Source: three-view drawing plus pictorial views. Frame: mm from the lowest corner of the part. Give positions to 0.01 mm unless a question says otherwise; leave off trailing zeros. Write each loop counter-clockwise with the first axis right and the second up, starting at its lowest first coordinate (ties: lowest second). Pieces come first, ordered by that corner, then holes. Notation, with made-up numbers: M 10.5,-17 L 28.5,-17 A28 ccw 28.5,21 Z; hole C 64,44.5 d2. An arc over 180 degrees is marked long. Return JSON: item names as keys, results as strings.
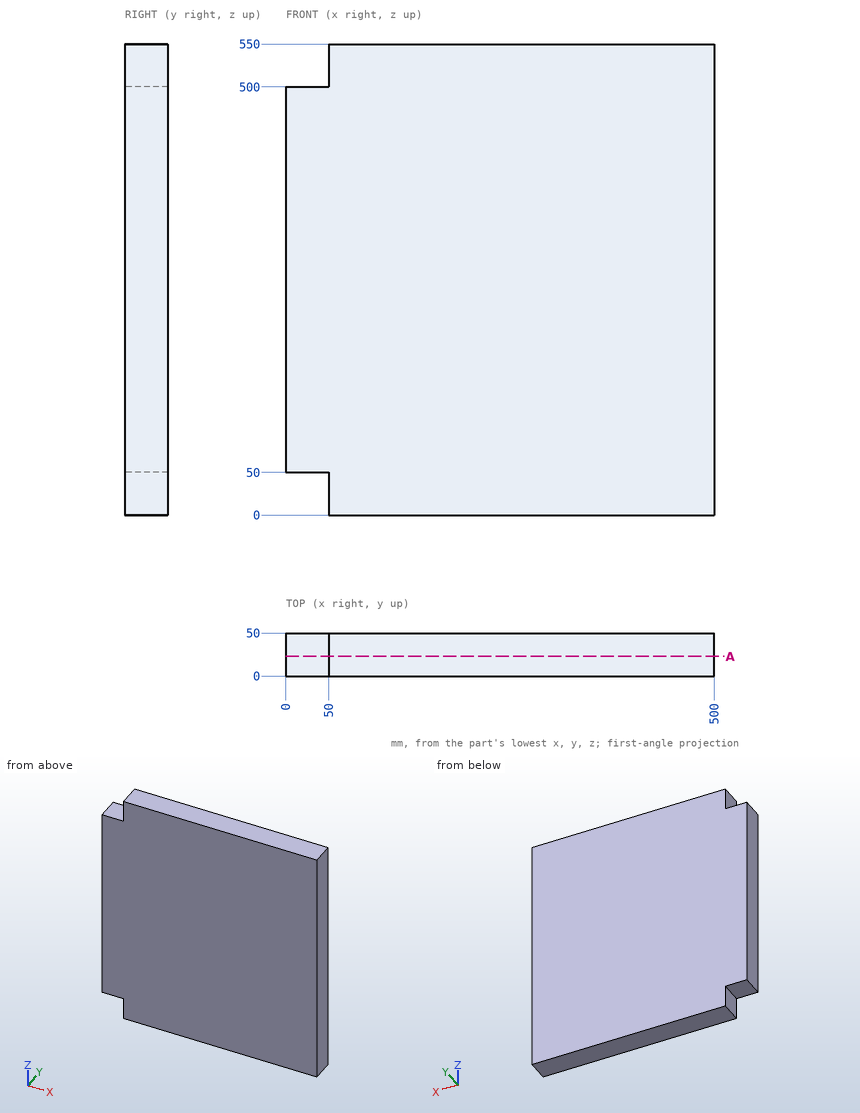
1) Contact query for flat-ended pins moving along their axis: pin 1 Ø12 at (x, z) = (430, 181.5) entering from -Y; pin 2 Ø25 at (x, y) = (26, 31.5) entering from -Z; pin 3 Ø25 at (y, z) = (35, 30) entering from -X. Output: stop coordinate, or through.
Numbers:
{"pin 1": "stops at y = 0", "pin 2": "stops at z = 50", "pin 3": "stops at x = 50"}
2) Cut plane A-A, the plane y = 23. Return the cut outline in (x, z).
Numbers:
{"outline": "M 0,50 L 50,50 L 50,0 L 500,0 L 500,550 L 50,550 L 50,500 L 0,500 Z"}
3) Line query: line 1 (X direction, y = 38, z = 519.5). Output: solid intervals per line, ascending. Write a range as [from, to].
Numbers:
{"line 1": "x = [50, 500]"}
